```python
from build123d import *

# Parameters (mm, degrees)
SKETCH1_W           = 170
SKETCH1_H           = 60
SKETCH1_R           = 4.5
SKETCH1_R_2         = 2.5
BOSS_EXTRUDE1_DEPTH = 6


with BuildPart() as part:
    # Sketch1 → Boss-Extrude1 (new body)
    with BuildSketch(Plane(origin=(0, 0, 0), x_dir=(-1, 0, 0), z_dir=(0, 0, -1))):
        with Locations((1, 5)):
            Rectangle(SKETCH1_W, SKETCH1_H)
        with Locations(Location((-30, 5, 0), (0, 0, 180))):
            Circle(SKETCH1_R, mode=Mode.SUBTRACT)
        with Locations(Location((-49, 5, 0), (0, 0, 180))):
            Circle(SKETCH1_R, mode=Mode.SUBTRACT)
        with Locations(Location((32, 5, 0), (0, 0, 180))):
            Circle(SKETCH1_R, mode=Mode.SUBTRACT)
        with Locations(Location((51, 5, 0), (0, 0, 180))):
            Circle(SKETCH1_R, mode=Mode.SUBTRACT)
        with Locations((79.445, 23.5)):
            Circle(SKETCH1_R_2, mode=Mode.SUBTRACT)
        with Locations((79.455, -13.5)):
            Circle(SKETCH1_R_2, mode=Mode.SUBTRACT)
        with Locations((-77.445, -13.5)):
            Circle(SKETCH1_R_2, mode=Mode.SUBTRACT)
        with Locations((-77.455, 23.5)):
            Circle(SKETCH1_R_2, mode=Mode.SUBTRACT)
    extrude(amount=-BOSS_EXTRUDE1_DEPTH)


solid = part.part
```
Verification items for the finished model (mm, model axes). Round coordinates to 2 decimals unless told otherwise and drop trailing zeros. Order: outer loops, then holes, each group sorted by start corner. A loop starts at its lowest first (then second) coordinate and runs counter-clockwise, first axis right, second up.
1) Cross-section at C-C, the plane x = 30. Record the cut outline in (y, z), plus the area to 3 significant figures.
Geometry says:
outline: (-25, 0) - (0.5, 0) - (0.5, 6) - (-25, 6) - close; (9.5, 0) - (35, 0) - (35, 6) - (9.5, 6) - close
area: 306 mm2
2) Cross-section at A-A, the plane y = 5. Record the cut outline in (x, z).
Geometry says:
outline: (-86, 0) - (-55.5, 0) - (-55.5, 6) - (-86, 6) - close; (-46.5, 0) - (-36.5, 0) - (-36.5, 6) - (-46.5, 6) - close; (-27.5, 0) - (25.5, 0) - (25.5, 6) - (-27.5, 6) - close; (34.5, 0) - (44.5, 0) - (44.5, 6) - (34.5, 6) - close; (53.5, 0) - (84, 0) - (84, 6) - (53.5, 6) - close
3) Material ranges on line 1 (Y direction, x = 30, z = 2.95); line 2 (X direction, y = 24, z = 5.4); line 3 (X direction, y = 21.5, z = 3.6) (3 decimals), recorded low to high.
Geometry says:
line 1: y = -25 to 0.5, 9.5 to 35
line 2: x = -86 to -81.89, -77 to 75.01, 79.9 to 84
line 3: x = -86 to -80.945, -77.945 to 75.955, 78.955 to 84
4) Draft check along X on faces 1 (the cylindrical face through (-76.947, 23.61, 2.958)), 2 (the flat face through (0, 5, 0)), 3 (the flat face through (84, 5, 3)), 4 (the cylindrical face through (76.1, 25.6, 3)). Enter one of: +X half, -X half, draft (parallel to the pull), parting line (faces both ways), or undercut.
Geometry says:
face 1: undercut
face 2: draft
face 3: +X half
face 4: undercut
5) Depth check by flat-ended pin: pin 1 (1 mm diameter, centred on x = -17, y = -14.5, fed in from -Z). Enter the tip coordinate at first touch or a pass-through.
Geometry says:
pin 1: stops at z = 0
6) Cross-section at D-D, the plane z = 3.35. Give the number of separate pieces and of enclosed holes in the cut face, plus the area to 3 significant figures.
Geometry says:
separate pieces: 1
enclosed holes: 8
area: 9,870 mm2
7) Cross-section at B-B, the plane y = 23.5. Record the cut outline in (x, z) (3 decimals).
Geometry says:
outline: (-86, 0) - (-81.945, 0) - (-81.945, 6) - (-86, 6) - close; (-76.945, 0) - (74.955, 0) - (74.955, 6) - (-76.945, 6) - close; (79.955, 0) - (84, 0) - (84, 6) - (79.955, 6) - close
